Read the model definition and answer for the solid it produces. Units are mm, in the model's axes. Round coordinates to 2 decimals unless told otherwise and drop trailing zeros. Loops run counter-clockwise (first coordinate to the right, second up) from the corner with the lowest first, then second, coordinate; pieces in that order, holes last. Notation, with made-up numbers: (28, 19.25) -> (82, 19.25) arc R24 cw to (82, 42.25) -> close; hole circle Ø2 at (63.25, 38). An arc over 180 degrees is marked (long way). Put each result on its own line as item: value.
from build123d import *

# Parameters (mm, degrees)
BOSS_EXTRUDE1_DEPTH   = 4
BOSS_EXTRUDE1_2_DEPTH = 4
SKETCH2_R             = 14
BOSS_EXTRUDE2_DEPTH   = 8.8


with BuildPart() as part:
    # Sketch1 → Boss-Extrude1 (new, symmetric)
    with BuildSketch(Plane(origin=(0, 0, 0), x_dir=(0, 0, -1), z_dir=(1, 0, 0))):
        Polygon((-8.001, 12), (-14.6685, 53.34), (-6.8453, 151.13), (-2.4892, 174.244), (0, 177.8), (3.7338, 174.244), (5.6007, 151.13), (12.0015, 53.34), (8.001, 12), align=None)
    extrude(amount=BOSS_EXTRUDE1_DEPTH, both=True)



with BuildPart() as body_2:
    # Sketch1 → Boss-Extrude1 2 (new, symmetric)
    with BuildSketch(Plane(origin=(0, 0, 0), x_dir=(0, 0, -1), z_dir=(1, 0, 0))):
        Polygon((-8.001, -12), (-14.6685, -53.34), (-6.8453, -151.13), (-2.4892, -174.244), (0, -177.8), (3.7338, -174.244), (5.6007, -151.13), (12.0015, -53.34), (8.001, -12), align=None)
    extrude(amount=BOSS_EXTRUDE1_2_DEPTH, both=True)


with BuildPart() as part_1:
    add(part.part)

    add(body_2.part)  # Boss-Extrude2 merges body 2
    # Sketch2 → Boss-Extrude2 (add, symmetric)
    with BuildSketch(Plane(origin=(0, 0, 0), x_dir=(0, 0, -1), z_dir=(1, 0, 0))):
        Circle(SKETCH2_R)
    extrude(amount=BOSS_EXTRUDE2_DEPTH, both=True)


solid = part_1.part
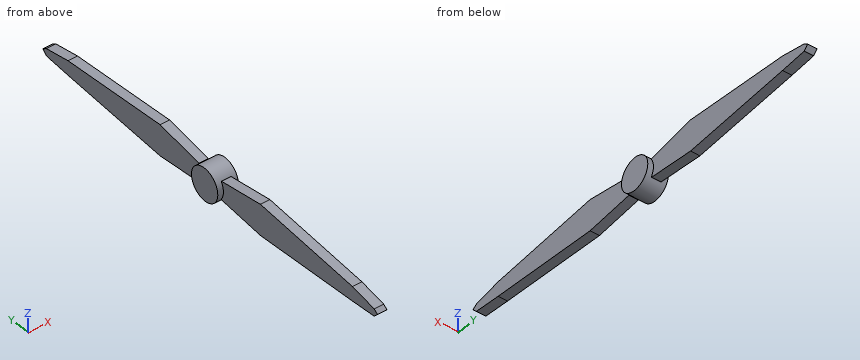
Item 1: The part is cut by section B-B (y = 0). Determine the outline of the cut face in (x, z).
Derived:
outline: (-8.8, -14) -> (8.8, -14) -> (8.8, 14) -> (-8.8, 14) -> close
Item 2: Flat-ended cylindrical pins translate along their axes: pin 1 Ø1 at (x, z) = (-6, -3.5) entering from -Y; pin 2 Ø12 at (y, z) = (-138, -3.5) entering from -X; pin 3 Ø2 at (x, y) = (-1, -13) entering from +Z. Find the tip coordinate at first contact, or state that the pin passes through.
Derived:
pin 1: stops at y = -13.67
pin 2: stops at x = -4
pin 3: stops at z = 8.32
Item 3: Find the intervals of material crossed by line 1 along X through (y, z) = (104, 10.25); line 2 along Z through (x, y) = (-0.5, -110); line 3 along Y through (x, z) = (-8, -9), in increasing order.
Derived:
line 1: x = -4 to 4
line 2: z = -8.29 to 10.14
line 3: y = -10.72 to 10.72
Item 4: The part is cut by section C-C (y = 102). Determine the outline of the cut face in (x, z), then the cut area to 3 significant figures.
Derived:
outline: (-4, -8.82) -> (4, -8.82) -> (4, 10.78) -> (-4, 10.78) -> close
area: 157 mm^2
Item 5: The part is cut by section A-A (x = -0.25). Determine the outline of the cut face in (y, z).
Derived:
outline: (-177.8, 0) -> (-174.24, -3.73) -> (-151.13, -5.6) -> (-53.34, -12) -> (-12, -8) -> (-12, -7.21) arc R14 ccw to (12, -7.21) -> (12, -8) -> (53.34, -12) -> (151.13, -5.6) -> (174.24, -3.73) -> (177.8, 0) -> (174.24, 2.49) -> (151.13, 6.85) -> (53.34, 14.67) -> (12, 8) -> (12, 7.21) arc R14 ccw to (-12, 7.21) -> (-12, 8) -> (-53.34, 14.67) -> (-151.13, 6.85) -> (-174.24, 2.49) -> close
